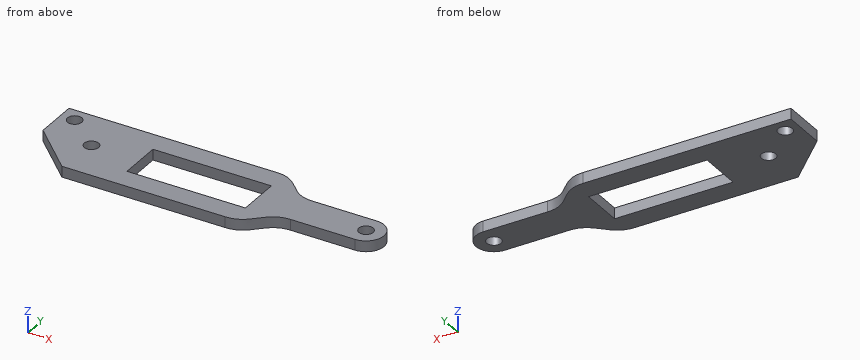
from build123d import *

# Parameters (mm, degrees)
ESQUISSE1_R        = 2
ESQUISSE1_W        = 33
ESQUISSE1_H        = 12
BOSS_EXTRU_1_DEPTH = 3


with BuildPart() as part:
    # Esquisse1 → Boss.-Extru.1 (new body)
    with BuildSketch(Plane.XY):
        with BuildLine():
            Line((-47.5, 12), (-47.5, 0))
            Line((-47.5, 0), (-35, -12))
            Line((-35, -12), (10.5, -12))
            add(Edge.make_bspline(
                [(10.5, -12), (17.5, -12), (17.5, -5), (24.5, -5)],
                knots=[0.5, 0.5, 0.5, 0.5, 1.5, 1.5, 1.5, 1.5], degree=3))
            Line((24.5, -5), (42.5, -5))
            ThreePointArc((42.5, -5), (47.5, 0), (42.5, 5))
            Line((42.5, 5), (24.5, 5))
            add(Edge.make_bspline(
                [(24.5, 5), (17.5, 5), (17.5, 12), (10.5, 12)],
                knots=[0, 0, 0, 0, 1, 1, 1, 1], degree=3))
            Line((10.5, 12), (-47.5, 12))
        make_face()
        with Locations((-34, 0)):
            Circle(ESQUISSE1_R, mode=Mode.SUBTRACT)
        with Locations((-4, 0)):
            Rectangle(ESQUISSE1_W, ESQUISSE1_H, mode=Mode.SUBTRACT)
        with Locations((-43.5, 8)):
            Circle(ESQUISSE1_R, mode=Mode.SUBTRACT)
        with Locations((42.5, 0)):
            Circle(ESQUISSE1_R, mode=Mode.SUBTRACT)
    extrude(amount=BOSS_EXTRU_1_DEPTH)


solid = part.part
Check sheet for the modelled part. Datum: model origin and axes. Units: mm. Coordinates: 2 decimals unless noted, no trailing zeros. Write each loop counter-clockwise with the first axis right and the second up, starting at its lowest first coordinate (ties: lowest second). Pieces come first, ordered by that corner, then holes.
Item 1: Cross-section at A-A on x = -43.5. Record the boundary of the cut face in (y, z).
Numbers:
outline: (-3.84, 0) - (6, 0) - (6, 3) - (-3.84, 3) - close; (10, 0) - (12, 0) - (12, 3) - (10, 3) - close
Item 2: Cross-section at C-C on z = 1. Count the separate pieces of the cut face and the enclosed holes in it, then the cut area to 3 significant figures.
Numbers:
separate pieces: 1
enclosed holes: 4
area: 1,340 mm2
Item 3: Depth check by flat-ended pin: pin 1 Ø4 at (x, y) = (30.5, 7.5) entering from -Z; pin 2 Ø1 at (y, z) = (1, 2) entering from +X; pin 3 Ø1.5 at (y, z) = (-2, 1) entering from -X; pin 4 Ø0.9 at (x, z) = (37, 2) entering from -Y. Enter the tip coordinate at first touch or a pass-through.
Numbers:
pin 1: passes through
pin 2: stops at x = 47.47
pin 3: stops at x = -46.2
pin 4: stops at y = -5
Item 4: Cross-section at B-B on x = -18.5. Record the boundary of the cut face in (y, z), then the cut area to 3 significant figures.
Numbers:
outline: (-12, 0) - (-6, 0) - (-6, 3) - (-12, 3) - close; (6, 0) - (12, 0) - (12, 3) - (6, 3) - close
area: 36.0 mm2
Item 5: Scan lines: probe 1 along Y at (x, z) = (42.5, 0.75); probe 2 along Y at (x, z) = (-12.5, 0.1); probe 3 along X at (y, z) = (1, 2.3). Record each from-to range of solid material in increasing order.
Numbers:
probe 1: y = -5 to -2, 2 to 5
probe 2: y = -12 to -6, 6 to 12
probe 3: x = -47.5 to -35.73, -32.27 to -20.5, 12.5 to 40.77, 44.23 to 47.4
